Part print with two shaded views. Sizes in mm from the minimum x, y, z corner. Coordinates: 2 decimals unless noted, no trailing zeros. Write each loop counter-clockwise with the first axis right and the second up, starting at its lowest first coordinate (ties: lowest second). Pieces come first, ordered by that corner, then holes. Notation, with made-up numbers: (-35.75, 9.25) - (-7.75, 9.25) arc R21 cw to (-7.75, 38.25) - close; hole circle Ø4 at (25.5, 7.5). An arc over 180 degrees is marked (long way). One line per question, with ' | ' between items. Start each with the question number.
1. Band-saw the part on C-C, the plane z = 3. Write the cut outline in (x, y).
2. Flat gauge pins, fed straight in: P1, Ø2, axis at y = 10, z = 15.5, coming from the -X side; P2, Ø1.5, axis at y = 2.5, z = 10.5, coming from the +X side; P3, Ø3, axis at y = 10, z = 7, coming from the +X side; P4, Ø5, axis at x = 5.5, z = 6.5, coming from the +Y side. Where does each tip first touch, or does it go through?
3. Band-saw the part on A-A, the plane x = 6.35. Write the cut outline in (y, z), then the cut area to 3 significant figures.
4. Two-plate mould, pull along Y, no slides. Class the marked faces 1, 2 and 3: +Y half, -Y half, draft (parallel to the pull), parting line (faces both ways), or undercut.
5. Probe line 1 (Y direction, x = 6.35, z = 4.5); line 2 (X direction, y = 8, z = 2.25); line 3 (Z direction, x = 0.75, y = 4.25). List the from-to ranges inside material, lowest first.
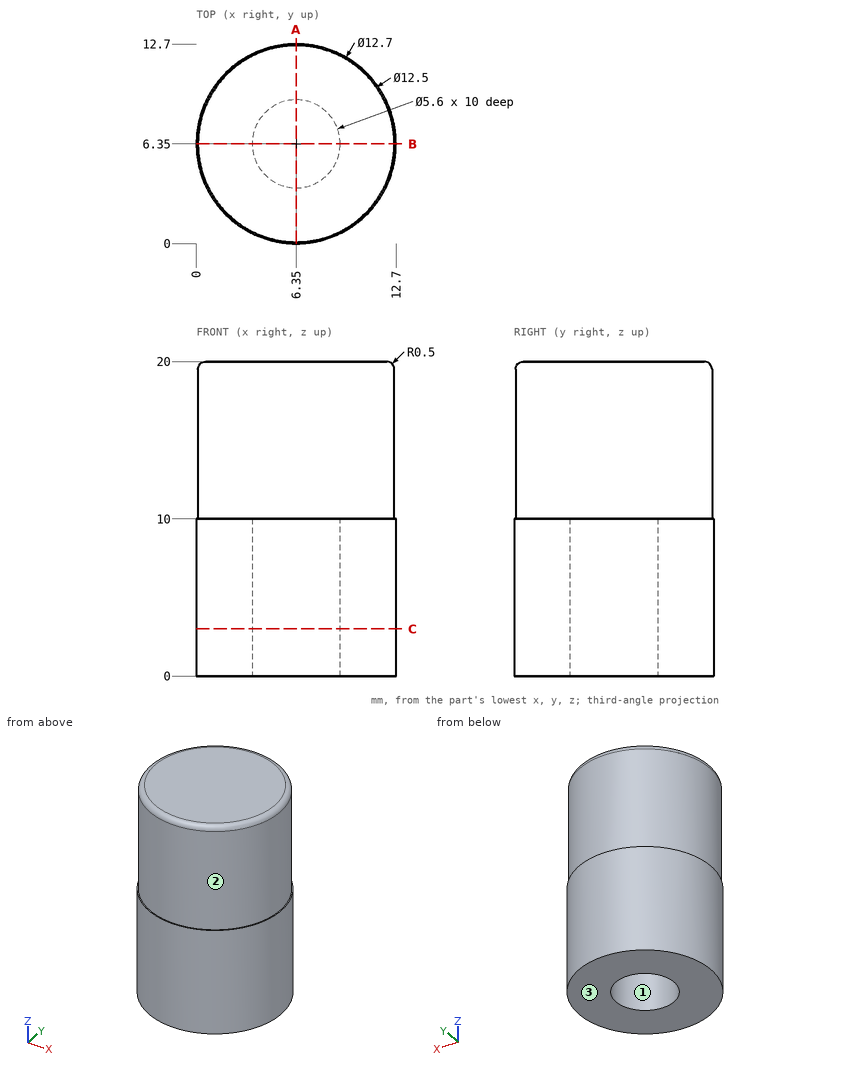
Filled in:
1) outline: circle Ø12.7 at (6.35, 6.35); hole circle Ø5.6 at (6.35, 6.35)
2) P1: stops at x = 0.69 | P2: stops at x = 11.78 | P3: stops at x = 12.32 | P4: stops at y = 12.7
3) outline: (0, 0) - (3.55, 0) - (3.55, 10) - (9.15, 10) - (9.15, 0) - (12.7, 0) - (12.7, 10) - (12.6, 10) - (12.6, 19.5) arc R0.5 ccw to (12.1, 20) - (0.6, 20) arc R0.5 ccw to (0.1, 19.5) - (0.1, 10) - (0, 10) - close | area: 196 mm²
4) face 1: undercut | face 2: parting line | face 3: draft
5) line 1: y = 0 to 3.55, 9.15 to 12.7 | line 2: x = 0.22 to 4.09, 8.61 to 12.48 | line 3: z = 0 to 19.94
